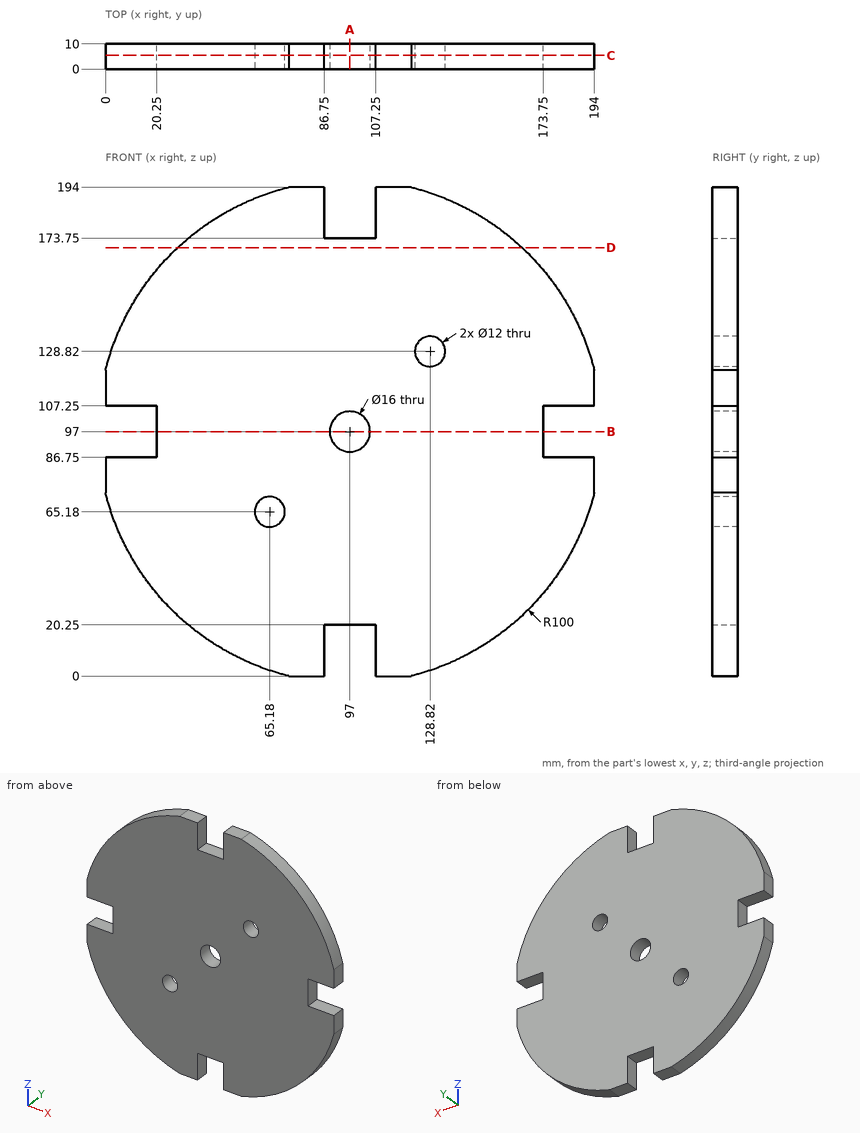
For this review, use the dimensioned drawing (mm, ordinates from the lowest corner) and the shaded views. Coordinates: 2 decimals unless noted, no trailing zeros. Write each loop counter-clockwise with the first axis right and the second up, starting at its lowest first coordinate (ties: lowest second). Pieces come first, ordered by that corner, then holes. Notation, with made-up numbers: (82, 36) - (132, 36) arc R22 ccw to (132, 63) - close; hole circle Ø1 at (32.5, 80). An arc over 180 degrees is marked (long way). Answer as a JSON object with one key per item and string values. Group by question number.
1. Add section C-C (y = 5.5). Give the boundary of the cut face in (x, z).
2. Clearance check with flat-ended pins moving along their axes: pin 1 Ø3 at (y, z) = (6.5, 98) entering from -X; pin 2 Ø3 at (y, z) = (6.5, 182) entering from -X (1 decimal); pin 3 Ø5 at (y, z) = (6, 14.5) entering from +X. State where each tip first meets the part, or that it passes through.
3. Add section B-B (z = 97). Give the boundary of the cut face in (x, y).
4. Add section A-A (x = 97). Give the boundary of the cut face in (y, z).
5. To check wall thickness, follow probe 1 along Z at (x, y) = (97, 7.5); probe 2 along X at (y, z) = (9.25, 63.5); probe 3 along Z at (x, y) = (128, 1). State the ranges of each line that lie inside material, in increasing order.
6. Add section D-D (z = 170). Give the boundary of the cut face in (x, y) (1 decimal).
Findings:
{
 "1": {"outline": "(0, 72.69) arc R100 ccw to (72.69, 0) - (86.75, 0) - (86.75, 20.25) - (107.25, 20.25) - (107.25, 0) - (121.31, 0) arc R100 ccw to (194, 72.69) - (194, 86.75) - (173.75, 86.75) - (173.75, 107.25) - (194, 107.25) - (194, 121.31) arc R100 ccw to (121.31, 194) - (107.25, 194) - (107.25, 173.75) - (86.75, 173.75) - (86.75, 194) - (72.69, 194) arc R100 ccw to (0, 121.31) - (0, 107.25) - (20.25, 107.25) - (20.25, 86.75) - (0, 86.75) - close; hole circle Ø12 at (65.18, 65.18); hole circle Ø16 at (97, 97); hole circle Ø12 at (128.82, 128.82)"},
 "2": {"pin 1": "x = 20.25", "pin 2": "x = 42", "pin 3": "x = 157"},
 "3": {"outline": "(20.25, 0) - (89, 0) - (89, 10) - (20.25, 10) - close; (105, 0) - (173.75, 0) - (173.75, 10) - (105, 10) - close"},
 "4": {"outline": "(0, 20.25) - (10, 20.25) - (10, 89) - (0, 89) - close; (0, 105) - (10, 105) - (10, 173.75) - (0, 173.75) - close"},
 "5": {"probe 1": "20.25 to 89, 105 to 173.75", "probe 2": "2.78 to 59.42, 70.94 to 191.22", "probe 3": "1.93 to 122.88, 134.76 to 192.07"},
 "6": {"outline": "(28.7, 0) - (165.3, 0) - (165.3, 10) - (28.7, 10) - close"}
}
